Autodesk Inventor part; units mm, degrees
ref_plane "РабПлоскость3" through (0, 7.615, 0) normal (0, 1, 0) x (-1, 0, 0)
ref_plane "YZ Plane" through (0, 0, 0) normal (1, 0, 0) x (0, 1, 0)
ref_plane "XY Plane" through (0, 0, 0) normal (0, 0, 1) x (1, 0, 0)
sketch "Эскиз4" plane through (0, 0, 0) normal (0, 0, 1) x (1, 0, 0)
  line L0 (-4.4, 7.615) -> (4.4, 7.615) construction
  line L1 (4.4, 7.615) -> (4.4, -7.615) construction
  line L2 (4.4, -7.615) -> (-4.4, -7.615) construction
  line L3 (-4.4, -7.615) -> (-4.4, 7.615) construction
  line L4 (-2.89, 7.615) -> (-2.89, -7.615) construction
  line L5 (2.89, 7.615) -> (2.89, -7.615) construction
  line L6 (-4.4, 6.105) -> (4.4, 6.105) construction
  line L7 (-4.4, -6.105) -> (4.4, -6.105) construction
  line L8 (-4.4, 5.175) -> (4.4, 5.175) construction
  line L9 (-4.4, -5.175) -> (4.4, -5.175) construction
  line L10 (-4.4, 4.987) -> (4.4, 4.987) construction
  line L11 (-4.4, -4.987) -> (4.4, -4.987) construction
  line L12 (-4.1, 7.615) -> (-4.1, -7.615) construction
  line L13 (4.1, 7.615) -> (4.1, -7.615) construction
  line L14 (-0.5, 7.615) -> (-0.5, -7.615) construction
  line L15 (0.5, 7.615) -> (0.5, -7.615) construction
  line L16 (-4.4, 4.32) -> (4.4, 4.32) construction
  line L17 (-4.4, -4.32) -> (4.4, -4.32) construction
  line L18 (-2.89, 7.615) -> (-4.4, 6.105)
  line L19 (-4.4, 6.105) -> (-4.4, 5.175)
  line L20 (-4.4, 5.175) -> (-4.1, 4.987)
  line L21 (-0.5, 4.987) -> (-4.1, 4.987)
  line L22 (-0.5, 4.32) -> (-0.5, 4.987)
  line L23 (-0.5, 4.32) -> (0.5, 4.32)
  line L24 (0.5, 4.32) -> (0.5, 4.987)
  line L25 (0.5, 4.987) -> (4.1, 4.987)
  line L26 (4.1, 4.987) -> (4.4, 5.175)
  line L27 (4.4, 5.175) -> (4.4, 6.105)
  line L28 (4.4, 6.105) -> (2.89, 7.615)
  line L29 (-2.89, 7.615) -> (2.89, 7.615)
  line L30 (-4.4, 0) -> (4.4, 0)
  point P0 (0, 0)
  point P1 (-4.4, 0)
  point P2 (0, 7.615)
  point P3 (0, 0)
  dimension "d17" = 8.8
  dimension "d18" = 15.23
  dimension "d19" = 5.78
  dimension "d20" = 2.89
  dimension "d21" = 12.21
  dimension "d22" = 6.105
  dimension "d23" = 10.35
  dimension "d24" = 5.175
  dimension "d25" = 9.974
  dimension "d26" = 4.987
  dimension "d27" = 0.3
  dimension "d28" = 0.3
  dimension "d29" = 0.5
  dimension "d30" = 1
  dimension "d31" = 8.64
  dimension "d32" = 4.32
  dimension "d33" = 8.8
  dimension "d34" = 7.615
revolve "Вращение2" add sketch "Эскиз4" angle 360 about axis through (-4.4, 0, 0) along (1, 0, 0)
ref_plane "РабПлоскость3" through (0, 7.615, 0) normal (0, 1, 0) x (-1, 0, 0)
sketch "Эскиз7" plane through (0, 7.615, 0) normal (0, 1, 0) x (-1, 0, 0)
  point P0 (0, 0)
ref_plane "Work Plane4" through (5.75, 0, 0) normal (1, 0, 0) x (0, 0, -1)
properties part number "CSW-1523"
For this review, take the finished solid that the model builds, in its own axes (mm). A direction names the side the tool comes from. Round coordinates to 2 decimals unless told otherwise and drop trailing zeros. Order: outer loops, then holes, each group sorted by start corner. A loop starts at its lowest first (then second) coordinate and runs counter-clockwise, first axis right, second up. Notation, with made-up numbers: (-37, -25) -> (-10, -25) arc R18 cw to (-10, -8) -> close; hole circle Ø2 at (42.5, 65.5). An arc over 180 degrees is marked (long way). Use a Markdown table: item, result.
Item 1: Machinability: for faces 4 (the flat face through (-4.4, -5, 3)), 5 (the cylindrical face through (-2.33, -1.08, 4.87)), 6 (the cylindrical face through (2.33, -1.08, -4.87)), which of the approach directions +Z, -Z, +X, -X, +Y, -Y give a long, thin tool a straight path to every point of the face, cutting with its end or side? Answer none if there is none.
Resolved:
| item | result |
|---|---|
| face 4 | +Z, -Z, -X, +Y, -Y |
| face 5 | -X |
| face 6 | +X |
Item 2: Take a section at C-C (x = 2). State the section outline as (y, z) points (3 decimals), plus the area to 3 significant figures.
Resolved:
| item | result |
|---|---|
| outline | circle Ø15.23 at (0, 0); hole circle Ø9.974 at (0, 0) |
| area | 104 mm² |
Item 3: Take a section at A-A (y = 0). State the section outline as (x, z) points (3 decimals).
Resolved:
| item | result |
|---|---|
| outline | (-4.4, -6.105) -> (-2.89, -7.615) -> (2.89, -7.615) -> (4.4, -6.105) -> (4.4, -5.175) -> (4.1, -4.987) -> (0.5, -4.987) -> (0.5, -4.32) -> (-0.5, -4.32) -> (-0.5, -4.987) -> (-4.1, -4.987) -> (-4.4, -5.175) -> close; (-4.4, 5.175) -> (-4.1, 4.987) -> (-0.5, 4.987) -> (-0.5, 4.32) -> (0.5, 4.32) -> (0.5, 4.987) -> (4.1, 4.987) -> (4.4, 5.175) -> (4.4, 6.105) -> (2.89, 7.615) -> (-2.89, 7.615) -> (-4.4, 6.105) -> close |
Item 4: For pin 1 (5 mm diameter, centred on y = -2, z = -1, fed in from -X); pin 2 (1.5 mm diameter, centred on x = 0.5, z = -4, fed in from +Y); pin 3 (5 mm diameter, centred on x = -1, z = -4.5, fed in from +Y), all flat-tipped, find the tip position at first contact; note any pin that passes through.
Resolved:
| item | result |
|---|---|
| pin 1 | stops at x = -0.5 |
| pin 2 | stops at y = 6.89 |
| pin 3 | stops at y = 7.35 |
Item 5: Draft analysis for pull direction Z (two halves, no side actions). For faces 1 (the cylindrical face through (0.04, -1.651, -7.434)), 2 (the cylindrical face through (0.01, 4.12, 1.3)), 3 (the flat face through (4.4, -5, 3)), state which applies: +Z half, -Z half, draft (parallel to the pull), parting line (faces both ways), or undercut.
Resolved:
| item | result |
|---|---|
| face 1 | parting line |
| face 2 | undercut |
| face 3 | draft |
Item 6: For line 1 along Z through (x, y) = (1.4, 0) (3 decimals); line 2 along Z through (x, y) = (-0.15, 0) (3 decimals); line 3 along Y through (x, z) = (1.75, 5.75), list the stretches that pass through material, from the lowest coordinate up. Write a range as [from, to].
Resolved:
| item | result |
|---|---|
| line 1 | z = [-7.615, -4.987], [4.987, 7.615] |
| line 2 | z = [-7.615, -4.32], [4.32, 7.615] |
| line 3 | y = [-4.99, 4.99] |
